Source: CAD feature listing. Evaluate the final solid. Frame: model axes, mm. A direction names the side the tool comes from. Coordinates: 2 decimals unless noted, no trailing zeros. Loops run counter-clockwise (first coordinate to the right, second up) from the corner with the lowest first, then second, coordinate; pieces in that order, holes last. Notation, with made-up numbers: M 7,84.5 L 56,84.5 A35 cw 56,121.5 Z; hole C 17,-11 d9. An arc over 180 degrees is marked long. Write each question's results on one line, items separated by ' | '. Start each with the question number.
from build123d import *

# Parameters (mm, degrees)
F0_R     = 18.808676083
F1_DEPTH = 69.1824834794
F2_R     = 12.9265710322
F3_DEPTH = 129.7349091619
F5_DEPTH = 129.6051889658
F6_R     = 16.6484962408
F7_DEPTH = 87.6426827163


with BuildPart() as f1:
    # F0 (on Front) → F1 (new body)
    with BuildSketch(Plane.XZ):
        with Locations((0, 77.7600631118)):
            Circle(F0_R)
    extrude(amount=F1_DEPTH)

    # F2 (on face) → F3 (cut)
    with BuildSketch(Plane.XZ.offset(69.1824834794)):
        with Locations((0, 77.7600631118)):
            Circle(F2_R)
    extrude(amount=-F3_DEPTH, mode=Mode.SUBTRACT)

    # F4 (on face) → F5 (cut)
    with BuildSketch(Plane.XZ.offset(69.1824834794)):
        with BuildLine():
            ThreePointArc((-12.9257110231, 77.6109551043), (0, 64.8334920796), (12.9257110231, 77.6109551043))
            ThreePointArc((12.9257110231, 77.6109551043), (0, 83.0086830497), (-12.9257110231, 77.6109551043))
        make_face()
        with BuildLine():
            ThreePointArc((-17.3048152374, 70.3905539291), (-2.8124051236, 46.8772133943), (18.1751909702, 64.8334920796))
            ThreePointArc((18.1751909702, 64.8334920796), (17.9562786853, 67.6458972031), (17.3048152374, 70.3905539291))
            ThreePointArc((17.3048152374, 70.3905539291), (0, 58.9513870288), (-17.3048152374, 70.3905539291))
        make_face()
    extrude(amount=-F5_DEPTH, mode=Mode.SUBTRACT)

    # F6 (on face) → F7 (cut)
    with BuildSketch(Plane.XZ.offset(69.1824834794)):
        with Locations((-1.8266138414, 64.963199413)):
            Circle(F6_R)
    extrude(amount=-F7_DEPTH, mode=Mode.SUBTRACT)


solid = f1.part
Item 1: Cut plane C-C (y = -49). Output: boundary loops of the cut face in (x, z).
Item 2: Line query: probe 1 along Z at (x, y) = (0, -38.5); probe 2 along X at (y, z) = (-17.5, 72.5); probe 3 along X at (y, z) = (-61, 86). Output: solid intervals per line, ascending.
Item 3: First-contact query: pin 1 Ø6 at (x, y) = (-7.5, -25) entering from -Z; pin 2 Ø12 at (y, z) = (-12.5, 81) entering from +X; pin 3 Ø10 at (y, z) = (-9.5, 87) entering from +X; pin 4 Ø6 at (x, y) = (4, -30) entering from -Z. Flat tips, straight axial feed; report the tip coordinate or a pass-through.
Item 4: Mould query, pull axis X, two halves, no side actions, for faces 1 (the cylindrical face through (2.14, -35.08, 90.51)), 2 (the cylindrical face through (3.203, -34.107, 96.294)), 3 (the flat face through (1, 0, 92)). Classes: +X half, -X half, draft (parallel to the pull), parting line (faces both ways), or undercut.
Item 5: Cut plane A-A (z = 73). Output: boundary loops of the cut face in (x, y).
Item 6: Cut plane B-B (x = 0). Output: boundary loops of the cut face in (y, z), then the cut area to 3 significant figures.
Item 7: Cut plane D-D (z = 83). Output: boundary loops of the cut face in (x, y).
Item 8: Access query for faces 4 (the cylindrical face through (14.025, -35.076, 70.051)), 5 (the flat face through (1, -69.182, 92)). Directions: +Z, -Z, +X, -X, +Y, -Y. A direction counts if a zero-diameter tool reaches every point of the face in a straight line with its end or side. Return the directions, or none.
Response values:
1) outline: M -17.44,70.73 A16.65 cw -12.92,77.38 A12.93 cw long 12.3,73.78 A16.65 cw 14.78,66.13 A18.81 ccw long Z
2) probe 1: z = 90.69 to 96.57 | probe 2: x = -18.06 to -16.67, 13.02 to 18.06 | probe 3: x = -16.91 to -9.96, 9.96 to 16.91
3) pin 1: stops at z = 85.3 | pin 2: stops at x = 18.81 | pin 3: stops at x = 18.32 | pin 4: stops at z = 88.63
4) face 1: undercut | face 2: parting line | face 3: draft
5) outline: M -18.2,-69.18 L -16.41,-69.18 L -16.41,0 L -18.2,0 Z; M 12.75,-69.18 L 18.2,-69.18 L 18.2,0 L 12.75,0 Z
6) outline: M -69.18,90.69 L 0,90.69 L 0,96.57 L -69.18,96.57 Z | area: 407 mm2
7) outline: M -18.06,-69.18 L -11.82,-69.18 L -11.82,0 L -18.06,0 Z; M 11.82,-69.18 L 18.06,-69.18 L 18.06,0 L 11.82,0 Z
8) face 4: -Z, +Y, -Y | face 5: +Z, -Z, +X, -X, -Y
